Design review of the part built by this model. Coordinates are the model's own, in mm. A direction names the side the tool comes from. Give positions to 0.01 mm unless a question says otherwise; leave off trailing zeros. Loops run counter-clockwise (first coordinate to the right, second up) from the corner with the lowest first, then second, coordinate; pieces in that order, holes last. Notation, with made-up numbers: M -23,22 L -13,22 A37 ccw -13,61 Z; hole C 27.5,-33.5 d4. An arc over 180 degrees is marked long. Use a Markdown table: item, result. Add a question column.
(1) Add section B-B, the plane z = -2.25. Give the boundary of the cut face in (x, y), then the cut area to 3 significant figures.
(2) Insertion check: pin 1 Ø3 at (x, y) = (-2, 0.5) entering from -Z; pin 2 Ø2 at (y, z) = (2.5, -7) entering from +X; pin 3 Ø1 at (y, z) = (-10, -1.5) entering from -X. Each pin has a flat end and moves straight along its axis. Give the tip position at first contact, or say it passes through.
(3) Add section D-D, the plane y = 7.5. Give the boundary of the cut face in (x, z), then the cut area to 3 significant figures.
(4) Draft analysis for pull direction X (two halves, no side actions). For faces 5 (the face through (6, 6, -15)), 6 (the face through (3.4, 0.1, 0)), 7 (the face through (-10.316, -7.91, 0.21)), state which applies: pulls with the +X half, pulls with the -X half, needs draft (parallel to the pull), parting line crosses it, or undercut.
(5) For faces 1 (the face through (3, -3, 15)), 2 (the face through (0, 2.625, 5)), 3 (the face through (-2.53, -1.95, 13.03)), 4 (the face through (-1.73, -7.81, -7.6)), list the 3-axis set-ups (+Z, -Z, +X, -X, +Y, -Y) from which the entire face can be reached by the end or side of a thin tool; tool diameter is ignored.
(6) For probe 1 along Y at (x, z) = (0, -4); probe 2 along Z at (x, y) = (-5.25, 1.5); probe 3 along X at (y, z) = (4.25, -12), list the stretches that pass through material, from the lowest coordinate up.
(7) Add section C-C, the plane x = 4. Give the boundary of the cut face in (y, z), then the cut area to 3 significant figures.
```python
from build123d import *

# Parameters (mm, degrees)
F0_R     = 13
F5_DEPTH = 15
F4_R     = 8
F6_DEPTH = 15
F3_R     = 3.2
F8_DEPTH = 4
F9_DEPTH = 11


with BuildPart() as f5:
    # F0 (on Top) → F5 (new body, symmetric)
    with BuildSketch(Plane.XY):
        Circle(F0_R)
    extrude(amount=F5_DEPTH, both=True)

    # F4 (on offset) → F6 (cut)
    with BuildSketch(Plane.XY.offset(-15)):
        Circle(F4_R)
    extrude(amount=F6_DEPTH, mode=Mode.SUBTRACT)

    # F3 (on offset) → F8 (cut)
    with BuildSketch(Plane.XY.offset(15)):
        with Locations((0.0063437128, 0)):
            Circle(F3_R)
    extrude(amount=-F8_DEPTH, mode=Mode.SUBTRACT)

    # F7 (on Top) → F9 (cut)
    with BuildSketch(Plane.XY):
        with BuildLine():
            Line((1.8168599408, 2.625), (-1.8433996128, 2.625))
            ThreePointArc((-1.8433996128, 2.625), (-0.013269836, -3.2022189551), (1.8168599408, 2.625))
        make_face()
    extrude(amount=F9_DEPTH, mode=Mode.SUBTRACT)


solid = f5.part
```
Established:
| question | item | result |
|---|---|---|
| 1 | outline | C 0,0 d26; hole C 0,0 d16 |
| 1 | area | 330 mm^2 |
| 2 | pin 1 | z = 0 |
| 2 | pin 2 | x = 12.91 |
| 2 | pin 3 | x = -8.87 |
| 3 | outline | M -10.62,-15 L -2.78,-15 L -2.78,0 L 2.78,0 L 2.78,-15 L 10.62,-15 L 10.62,15 L -10.62,15 Z |
| 3 | area | 554 mm^2 |
| 4 | face 5 | needs draft |
| 4 | face 6 | undercut |
| 4 | face 7 | parting line crosses it |
| 5 | face 1 | +Z, +X, -X, +Y, -Y |
| 5 | face 2 | +Z, -Z |
| 5 | face 3 | +Z |
| 5 | face 4 | -Z |
| 6 | probe 1 | -13 to -8, 8 to 13 |
| 6 | probe 2 | 0 to 15 |
| 6 | probe 3 | -12.29 to -6.78, 6.78 to 12.29 |
| 7 | outline | M -12.37,-15 L -6.93,-15 L -6.93,0 L 6.93,0 L 6.93,-15 L 12.37,-15 L 12.37,15 L -12.37,15 Z |
| 7 | area | 534 mm^2 |
